The model under review builds one solid part; all positions refer to its coordinate system, in mm. A direction names the side the tool comes from. Coordinates: 2 decimals unless noted, no trailing zeros. Loops run counter-clockwise (first coordinate to the right, second up) from the corner with the lowest first, then second, coordinate; pieces in that order, holes last. Notation, with made-up numbers: M 42.25,4.5 L 94.25,4.5 A26 ccw 94.25,39.5 Z; hole C 24,26.5 d2. An arc over 180 degrees is marked long. Write item = value, one per line. Start each with the question number.
Q1. We need section B-B on y = -31. Give the boundary of the cut face in (x, z).
Q2. Clearance check with flat-ended pins moving along their axes: pin 1 Ø4 at (x, y) = (97.5, -7) entering from +Z; pin 2 Ø1 at (y, z) = (-19, 49) entering from +X; pin 3 Ø6 at (x, y) = (232.5, -5) entering from +Z; pin 4 Ø7 at (x, z) = (10.16, 12.7) entering from +Y. State where each tip first meets the part, or that it passes through.
Q3. We need section A-A on z = 59. Give the boundary of the cut face in (x, y).
Q4. We need section C-C on x = 137. Give the boundary of the cut face in (y, z), and give its area (3 significant figures).
Q5. Wall thickness on probe 1 along Z at (x, y) = (10.16, -29); probe 2 along Z at (x, y) = (47, -27); probe 3 along X at (y, z) = (-26.5, 47.5): over which ranges is each line inside the solid? List them lowest first.
Q6. For faces 5 (the face through (87, -19, 25.4)), 6 (the face through (140, 0, 18)), 7 (the face through (195.3, -18.78, 53.04)), list the 3-axis set-ups (+Z, -Z, +X, -X, +Y, -Y) from which the entire face can be reached by the end or side of a thin tool; tool diameter is ignored.
Q7. Mouldability with a two-part tool opening along X and no side actions: class faces 1 (the face through (180.441, -18.783, 49.535)), 2 (the face through (264.09, -18.78, 18.63)), 3 (the face through (140, -38.1, 18)), 4 (the face through (195.217, -18.783, 70.757)) as released by +X, released by -X, zero draft, split by the parting line, or undercut.
from build123d import *

# Parameters (mm, degrees)
F1_DEPTH = 38.1
F3_DEPTH = 50.8
F4_R     = 5.08


with BuildPart() as f1:
    # F0 (on Front) → F1 (new body)
    with BuildSketch(Plane.XZ):
        with BuildLine():
            Line((0, 25.4), (0, 0))
            Line((0, 0), (203.2, 0))
            ThreePointArc((203.2, 0), (264.847349, 19.147038), (304.8, 69.85))
            ThreePointArc((304.8, 69.85), (252.294174, 32.367952), (187.784361, 32.86784))
            Line((187.784361, 32.86784), (201.084143, 68.571143))
            Line((201.084143, 68.571143), (189.183042, 73.004403))
            Line((189.183042, 73.004403), (171.45, 25.4))
            Line((171.45, 25.4), (0, 25.4))
        make_face()
    extrude(amount=F1_DEPTH)

    # F2 (on face) → F3 (cut)
    with BuildSketch(Plane.XZ.offset(38.1)):
        with BuildLine():
            ThreePointArc((13.97, 12.7), (7.465923, 15.394077), (10.16, 8.89))
            ThreePointArc((10.16, 8.89), (12.854077, 10.005923), (13.97, 12.7))
        make_face()
    extrude(amount=-F3_DEPTH, mode=Mode.SUBTRACT)

    # F4
    f4_edges = [f1.edges().sort_by_distance(p)[0] for p in [
        (187.784361, -19.05, 32.86784),
    ]]
    fillet(f4_edges, radius=F4_R)


solid = f1.part
Returned:
q1.outline = M 0,0 L 203.2,0 A108.82 ccw 304.8,69.85 A104.48 cw 193.08,31.26 A5.08 cw 189.67,37.93 L 201.08,68.57 L 189.18,73 L 171.45,25.4 L 0,25.4 Z; hole C 10.16,12.7 d7.62
q2.pin_1 = 25.4
q2.pin_2 = 294.43
q2.pin_3 = 28.55
q2.pin_4 = through
q3.outline = M 183.97,-38.1 L 197.52,-38.1 L 197.52,0 L 183.97,0 Z; M 295.56,-38.1 L 299.94,-38.1 L 299.94,0 L 295.56,0 Z
q4.outline = M -38.1,0 L 0,0 L 0,25.4 L -38.1,25.4 Z
q4.area = 968 mm^2
q5.probe_1 = 0 to 8.89, 16.51 to 25.4
q5.probe_2 = 0 to 25.4
q5.probe_3 = 179.68 to 193.23, 282.27 to 293.1
q6.face_5 = +Z, -X, +Y, -Y
q6.face_6 = +Z, -Z, +X, -X, +Y
q6.face_7 = +Y, -Y
q7.face_1 = released by -X
q7.face_2 = released by +X
q7.face_3 = zero draft
q7.face_4 = undercut
